Verification items for the finished model (mm, model axes). Face numbers are marked on the shaded views. A direction names the side the tool comes from. Round coordinates to 2 decimals unless told otherwise and drop trailing zeros. Write each loop counter-clockwise with the first axis right and the second up, starting at its lowest first coordinate (ties: lowest second). Pieces come first, ordered by that corner, then holes. Notation, with made-up numbers: (18.25, 85.25) - (53.25, 85.25) arc R25 ccw to (53.25, 124.25) - close; hole circle Ø3 at (47.25, 72). An arc over 180 degrees is marked (long way). Answer as a JSON object with one key per item and string values.
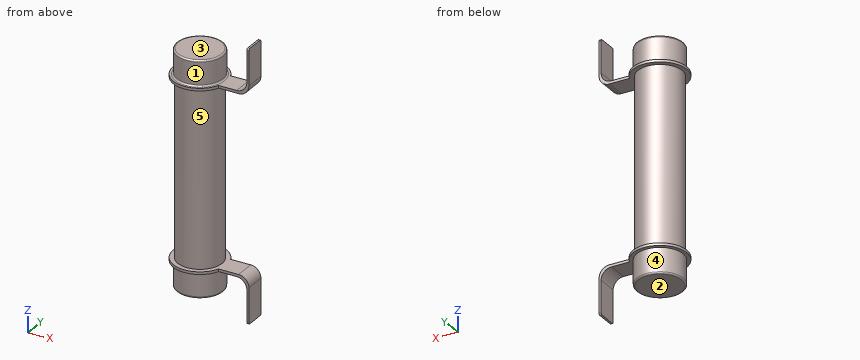
```python
from build123d import *

# Parameters (mm, degrees)
SKETCH1_R           = 4.3
BOSS_EXTRUDE1_DEPTH = 22.665
SKETCH2_R           = 4.5
SKETCH2_R_2         = 4.3
BOSS_EXTRUDE2_DEPTH = 5.43
SKETCH3_R           = 5.2
SKETCH3_R_2         = 4.5
BOSS_EXTRUDE3_DEPTH = 0.5
SKETCH5_W           = 9
SKETCH5_H           = 4
BOSS_EXTRUDE4_DEPTH = 0.4
SKETCH6_W           = 0.5
SKETCH6_H           = 4
BOSS_EXTRUDE5_DEPTH = 5.5
SKETCH7_W           = 9
SKETCH7_H           = 4
BOSS_EXTRUDE6_DEPTH = 0.4
SKETCH8_W           = 0.5
SKETCH8_H           = 4
BOSS_EXTRUDE7_DEPTH = 5.5
FILLET2_R           = 2
FILLET3_R           = 0.3


with BuildPart() as part:
    # Sketch1 → Boss-Extrude1 (new body, symmetric)
    with BuildSketch(Plane.XY):
        Circle(SKETCH1_R)
    extrude(amount=BOSS_EXTRUDE1_DEPTH, both=True)

    # Sketch2 → Boss-Extrude2 (add)
    with BuildSketch(Plane.XY.offset(22.665)):
        Circle(SKETCH2_R)
        Circle(SKETCH2_R_2, mode=Mode.SUBTRACT)
    boss_extrude2 = extrude(amount=-BOSS_EXTRUDE2_DEPTH)

    # Sketch3 → Boss-Extrude3 (add)
    with BuildSketch(Plane.XY.offset(17.235)):
        Circle(SKETCH3_R)
        Circle(SKETCH3_R_2, mode=Mode.SUBTRACT)
    boss_extrude3 = extrude(amount=BOSS_EXTRUDE3_DEPTH)

    # Mirror1: Boss-Extrude2, Boss-Extrude3 across plane
    add(boss_extrude2.mirror(Plane.XY))
    add(boss_extrude3.mirror(Plane.XY))



with BuildPart() as body_2:
    # Sketch5 → Boss-Extrude4 (new body)
    with BuildSketch(Plane(origin=(10.7, 0, 0), x_dir=(0, 0, -1), z_dir=(1, 0, 0))):
        with Locations((21.735, 0)):
            Rectangle(SKETCH5_W, SKETCH5_H)
    extrude(amount=-BOSS_EXTRUDE4_DEPTH)


with BuildPart() as part_1:
    add(part.part)

    add(body_2.part)  # Boss-Extrude5 merges body 2
    # Sketch6 → Boss-Extrude5 (add)
    with BuildSketch(Plane.ZY.offset(-10.3)):
        with Locations((-17.485, 0)):
            Rectangle(SKETCH6_W, SKETCH6_H)
    extrude(amount=BOSS_EXTRUDE5_DEPTH)



with BuildPart() as body_2_2:
    # Sketch7 → Boss-Extrude6 (new body)
    with BuildSketch(Plane(origin=(10.7, 0, 0), x_dir=(0, 0, -1), z_dir=(1, 0, 0))):
        with Locations((-21.735, 0)):
            Rectangle(SKETCH7_W, SKETCH7_H)
    extrude(amount=-BOSS_EXTRUDE6_DEPTH)


with BuildPart() as part_2:
    add(part_1.part)

    add(body_2_2.part)  # Boss-Extrude7 merges body 2 2
    # Sketch8 → Boss-Extrude7 (add)
    with BuildSketch(Plane.ZY.offset(-10.3)):
        with Locations((17.485, 0)):
            Rectangle(SKETCH8_W, SKETCH8_H)
    extrude(amount=BOSS_EXTRUDE7_DEPTH)

    # Fillet2
    fillet2_edges = [part_2.edges().sort_by_distance(p)[0] for p in [
        (10.3, 0, -17.735),
        (10.7, 0, -17.235),
        (10.3, 0, 17.735),
        (10.7, 0, 17.235),
    ]]
    fillet(fillet2_edges, radius=FILLET2_R)

    # Fillet3
    fillet3_edges = [part_2.edges().sort_by_distance(p)[0] for p in [
        (-4.5, 0, 17.735),
        (-4.5, 0, -22.665),
        (10.5, 2, -26.235),
        (10.5, -2, -26.235),
        (10.5, -2, 26.235),
        (10.5, 2, 26.235),
        (-4.5, 0, 22.665),
    ]]
    fillet(fillet3_edges, radius=FILLET3_R)


solid = part_2.part
```
Q1. Set-up check for the marked faces 1 and 2: record each of +Z, -Z, +X, -X, +Y, -Y from which the full face is reachable in a straight line by a thin tool's end or side.
Geometry check:
{"face 1": "+Z", "face 2": "-Z, -X, +Y, -Y"}
Q2. Section check C-C, the plane x = 9.25. Record the cut outline in (y, z), then the cut area to 3 significant figures.
Geometry check:
{"outline": "(-2, -17.98) - (2, -17.98) - (2, -17.31) - (-2, -17.31) - close; (-2, 17.31) - (2, 17.31) - (2, 17.98) - (-2, 17.98) - close", "area": "5.30 mm2"}
Q3. Section check D-D, the plane z = 23.5. Record the cut outline in (x, y), then the cut area to 3 significant figures.
Geometry check:
{"outline": "(10.3, -2) - (10.7, -2) - (10.7, 2) - (10.3, 2) - close", "area": "1.60 mm2"}
Q4. Section check A-A, the plane x = 0. Record the cut outline in (y, z) (3 decimals), then the cut area to 3 significant figures.
Geometry check:
{"outline": "(-5.2, -17.735) - (-4.5, -17.735) - (-4.5, -22.365) arc R0.3 ccw to (-4.2, -22.665) - (4.2, -22.665) arc R0.3 ccw to (4.5, -22.365) - (4.5, -17.735) - (5.2, -17.735) - (5.2, -17.235) - (4.3, -17.235) - (4.3, 17.235) - (5.2, 17.235) - (5.2, 17.735) - (4.8, 17.735) arc R0.3 cw to (4.5, 18.035) - (4.5, 22.365) arc R0.3 ccw to (4.2, 22.665) - (-4.2, 22.665) arc R0.3 ccw to (-4.5, 22.365) - (-4.5, 18.035) arc R0.3 cw to (-4.8, 17.735) - (-5.2, 17.735) - (-5.2, 17.235) - (-4.3, 17.235) - (-4.3, -17.235) - (-5.2, -17.235) - close", "area": "396 mm2"}
Q5. Gauge pin test, flat ends, axial feed: P1, Ø3, axis at y = 0.5, z = -23.5, coming from the -X side; P2, Ø4.5, axis at x = 7.5, z = 22, coming from the -Y side; P3, Ø3, axis at x = -3.5, z = 1.5, coming from the +Y side; P4, Ø1, axis at y = 1.5, z = 6.5, coming from the +X side. Record the tip position at first contact, or that the pin passes through.
Geometry check:
{"P1": "stops at x = -4.5", "P2": "passes through", "P3": "stops at y = 3.81", "P4": "stops at x = 4.18"}
Q6. Release check for a two-part mould opening along X. For the marked faces 3, 4 and 5 record: released by +X, released by -X, zero draft, split by the parting line, or undercut.
Geometry check:
{"face 3": "zero draft", "face 4": "undercut", "face 5": "split by the parting line"}
Q7. Material ranges on line 1 along Z through (x, y) = (3.75, 3.25) (3 decimals); line 2 along Z through (x, y) = (1.25, -4.5) (3 decimals); line 3 along Z through (x, y) = (0.75, 3.5) (3 decimals), recorded low to high. Write a range as [from, to].
Geometry check:
{"line 1": "z = [-17.735, -17.235], [17.235, 17.735]", "line 2": "z = [-17.735, -17.235], [17.235, 17.764]", "line 3": "z = [-22.665, 22.665]"}
